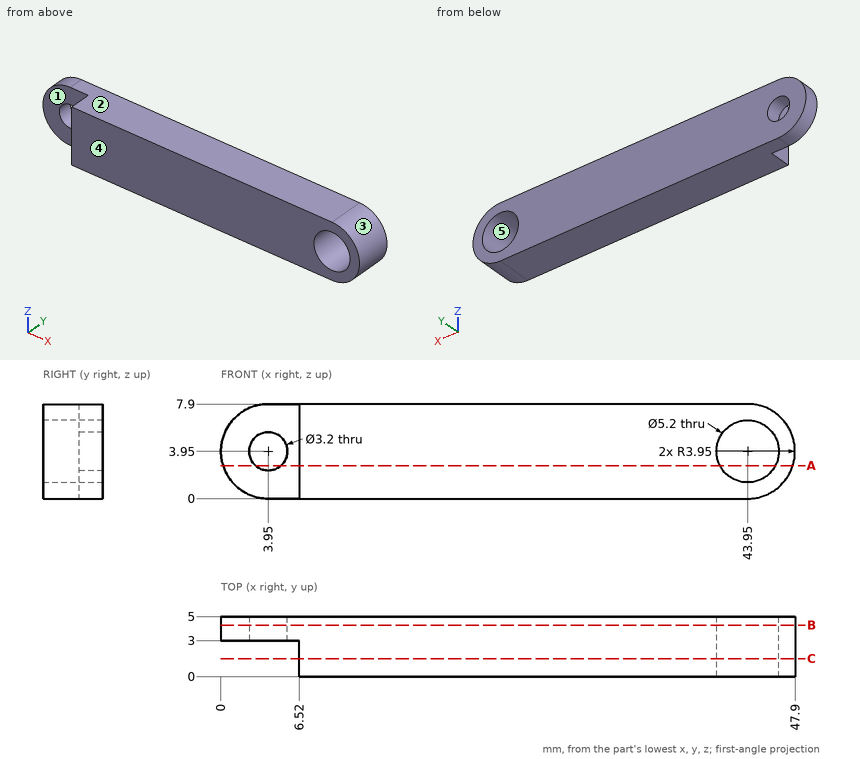
Drawing for the job (mm, zero at the part's lowest x, y, z). A direction names the side the tool comes from. Round coordinates to 2 decimals unless told otherwise and drop trailing zeros. Write each loop counter-clockwise with the first axis right and the second up, starting at its lowest first coordinate (ties: lowest second). Pieces come first, ordered by that corner, then holes. Notation, with made-up numbers: (-1.5, 58) - (38.5, 58) arc R18 cw to (38.5, 79) - close; hole circle Ø10 at (11, 80). An arc over 180 degrees is marked (long way). Write item = value, one per line. Start each with the question number.
Q1. Band-saw the part on C-C (y = 1.5). Give the cut face in (x, z).
Q2. Drop flat-ended pins along their axis: pin 1 (3.5 mm diameter, centred on x = 3.95, z = 3.95, fed in from -Y); pin 2 (1.5 mm diameter, centred on y = 2, z = 5, fed in from -X). Give the stop position or say it passes through.
Q3. Probe L1, parallel to X at y = 4, z = 4; L2, parallel to Z at x = 3.95, y = 3.45; L3, parallel to Z at x = 43.95, y = 1.55. List the from-to ranges inside material, lowest first. Write a range as from..to.
Q4. Which spindle directions (+Z, -Z, +X, -X, +Y, -Y) get a long thin tool onto all of the face, cutting with end or side? Do the marked faces 1 and 2. Say none if no direction does.
Q5. Band-saw the part on B-B (y = 4.3). Give the cut face in (x, z), then the cut area to 3 significant figures.
Q6. Mould opens along X. For the marked faces 3, 4 and 5 say: pulls with the +X half, pulls with the -X half, needs draft (parallel to the pull), parting line crosses it, or undercut.
Q7. Band-saw the part on A-A (z = 2.75). Give the cut face in (x, y).
Answers below:
q1.outline = (6.52, 0) - (43.95, 0) arc R3.95 ccw to (43.95, 7.9) - (6.52, 7.9) - close; hole circle Ø5.2 at (43.95, 3.95)
q2.pin_1 = 3
q2.pin_2 = 6.52
q3.L1 = 0..2.35, 5.55..41.35, 46.55..47.9
q3.L2 = 0..2.35, 5.55..7.9
q3.L3 = 0..1.35, 6.55..7.9
q4.face_1 = +Z, -Z, -X, -Y
q4.face_2 = +Z, +X, -X, +Y, -Y
q5.outline = (3.95, 0) - (43.95, 0) arc R3.95 ccw to (43.95, 7.9) - (3.95, 7.9) arc R3.95 ccw to start; hole circle Ø3.2 at (3.95, 3.95); hole circle Ø5.2 at (43.95, 3.95)
q5.area = 336 mm2
q6.face_3 = pulls with the +X half
q6.face_4 = needs draft
q6.face_5 = undercut
q7.outline = (0.19, 3) - (2.89, 3) - (2.89, 5) - (0.19, 5) - close; (5.01, 3) - (6.52, 3) - (6.52, 0) - (41.64, 0) - (41.64, 5) - (5.01, 5) - close; (46.26, 0) - (47.71, 0) - (47.71, 5) - (46.26, 5) - close
